Input: part model. Units: mm. Frame: model coordinates. A direction names the side the tool comes from. Round coordinates to 2 decimals unless told otherwise and drop trailing zeros. Write each loop counter-clockwise with the first axis right and the second up, starting at its lowest first coordinate (ties: lowest second). Pieces come first, ordered by that corner, then holes. Notation, with made-up numbers: (-22, 36.25) - (-10, 36.25) arc R15 cw to (-10, 65.25) - close; hole circle Ø6 at (5, -24.5). An arc over 180 degrees is marked (long way). Use one line per item in the form item = value.
```python
from build123d import *


with BuildPart() as f1:
    # F0 (on Front) → F1 (revolve)
    with BuildSketch(Plane.XZ):
        with BuildLine():
            Line((-9.624976, 4.035722), (0, 4.035722))
            Line((0, 4.035722), (0, 7.035722))
            Line((0, 7.035722), (-8.861714, 7.035722))
            ThreePointArc((-8.861714, 7.035722), (-10.481633, 8.559734), (-11.393906, 10.588161))
            Line((-11.393906, 10.588161), (-11.393906, 65.143411))
            ThreePointArc((-11.393906, 65.143411), (-9.78004, 71.654474), (-6.355783, 77.422746))
            ThreePointArc((-6.355783, 77.422746), (-4.858919, 83.721432), (-4.308291, 90.172079))
            Line((-4.308291, 90.172079), (-2.414047, 113.346809))
            Line((-2.414047, 113.346809), (-5.404075, 113.591207))
            Line((-5.404075, 113.591207), (-7.30709, 90.309181))
            ThreePointArc((-7.30709, 90.309181), (-7.771101, 84.515665), (-9.054899, 78.847156))
            ThreePointArc((-9.054899, 78.847156), (-12.694503, 72.447425), (-14.393906, 65.283954))
            Line((-14.393906, 65.283954), (-14.393906, 10.28396))
            ThreePointArc((-14.393906, 10.28396), (-12.756039, 6.590004), (-9.624976, 4.035722))
        make_face()
    revolve(axis=Axis((0, 0, 69.837436), (0, 0, 1)))


solid = f1.part
```
(1) Access query for faces 1 (the face through (-1.2, 2.308, 113.362)), 2 (the face through (2.47, 11.123, 38.248)). Directions: +Z, -Z, +X, -X, +Y, -Y. A direction counts if a zero-diameter tool reaches every point of the face in a straight line with its end or side. Return the directions, or none.
Derived:
face_1 = +Z
face_2 = none
(2) Cut plane A-A on z = 57.5. Output: boundary loops of the cut face in (x, y), then the cut area to 3 significant figures.
Derived:
outline = circle Ø28.79 at (0, 0); hole circle Ø22.79 at (0, 0)
area = 243 mm^2
(3) Draft query along Z for faces 3 (the face through (0, 0, 4.036)), 4 (the face through (5.05, 3.88, 101.79)), 5 (the face through (0, 0, 7.036)). Return one class per face: released by +Z, released by -Z, zero draft, split by the parting line, or undercut.
Derived:
face_3 = released by -Z
face_4 = released by +Z
face_5 = undercut
(4) First-contact query: pin 1 Ø2 at (y, z) = (1, 49) entering from +X; pin 2 Ø1 at (y, z) = (-0.5, 70.5) entering from +X. Flat tips, straight axial feed; report the tip coordinate or a pass-through.
Derived:
pin_1 = 14.39
pin_2 = 13.51
(5) Material intervals for L1, parallel to X at y = 0, z = 22.5; L2, parallel to X at y = 9.5, z = 50, sorted ascending.
Derived:
L1 = -14.39 to -11.39, 11.39 to 14.39
L2 = -10.81 to -6.29, 6.29 to 10.81
